from build123d import *

# Parameters (mm, degrees)
SKETCH1_R           = 17.5
BOSS_EXTRUDE1_DEPTH = 20
SKETCH2_R           = 21.5
BOSS_EXTRUDE2_DEPTH = 3
SKETCH3_W           = 19
SKETCH3_H           = 8.5
CUT_EXTRUDE3_DEPTH  = 23
FILLET11_R          = 4
FILLET12_R          = 4


with BuildPart() as part:
    # Sketch1 → Boss-Extrude1 (new body)
    with BuildSketch(Plane(origin=(0, 0, 0), x_dir=(1, 0, 0), z_dir=(0, 1, 0))):
        with Locations(Location((0, 0, 0), (0, 0, 270))):
            Circle(SKETCH1_R)
    extrude(amount=BOSS_EXTRUDE1_DEPTH)

    # Sketch2 → Boss-Extrude2 (add)
    with BuildSketch(Plane(origin=(0, 20, 0), x_dir=(1, 0, 0), z_dir=(0, 1, 0))):
        with Locations(Location((0, 0, 0), (0, 0, 270))):
            Circle(SKETCH2_R)
    extrude(amount=BOSS_EXTRUDE2_DEPTH)

    # Sketch3 → Cut-Extrude3 (cut)
    with BuildSketch(Plane(origin=(0, 23, 0), x_dir=(1, 0, 0), z_dir=(0, 1, 0))):
        with Locations((0, 0.083811037)):
            Rectangle(SKETCH3_W, SKETCH3_H)
        with Locations((0, 10.083811037)):
            Rectangle(SKETCH3_W, SKETCH3_H)
        with Locations((0, -9.916188963)):
            Rectangle(SKETCH3_W, SKETCH3_H)
    extrude(amount=-CUT_EXTRUDE3_DEPTH, mode=Mode.SUBTRACT)

    # Fillet11
    fillet11_edges = [part.edges().sort_by_distance(p)[0] for p in [
        (9.5, 11.5, 4.166188963),
        (-9.5, 11.5, 4.166188963),
        (-9.5, 11.5, -4.333811037),
        (9.5, 11.5, -4.333811037),
        (9.5, 11.5, 14.166188963),
        (-9.5, 11.5, 14.166188963),
        (-9.5, 11.5, 5.666188963),
        (9.5, 11.5, 5.666188963),
    ]]
    fillet(fillet11_edges, radius=FILLET11_R)

    # Fillet12
    fillet12_edges = [part.edges().sort_by_distance(p)[0] for p in [
        (9.5, 11.5, -14.333811037),
        (9.5, 11.5, -5.833811037),
        (-9.5, 11.5, -5.833811037),
        (-9.5, 11.5, -14.333811037),
    ]]
    fillet(fillet12_edges, radius=FILLET12_R)


solid = part.part
Read the model definition and answer for the solid it produces. Units are mm, in the model's axes. A direction names the side the tool comes from. Coordinates: 2 decimals unless noted, no trailing zeros. Order: outer loops, then holes, each group sorted by start corner. A loop starts at its lowest first (then second) coordinate and runs counter-clockwise, first axis right, second up. Notation, with made-up numbers: (18, -9.5) - (36, -9.5) arc R30 ccw to (36, 25.5) - close; hole circle Ø6 at (85, 86.5). An arc over 180 degrees is marked (long way). Use one line per item in the form item = value.
(1) Section C-C, the plane z = -11.5 is taken. Give the vertices of the cut face in (x, y).
Computed values:
outline = (-18.17, 20) - (-13.19, 20) - (-13.19, 0) - (-9.33, 0) - (-9.33, 23) - (-18.17, 23) - close; (9.33, 0) - (13.19, 0) - (13.19, 20) - (18.17, 20) - (18.17, 23) - (9.33, 23) - close
(2) Given pin 1 Ø3.5 at (x, y) = (-2, 11.5) entering from +Z; pin 2 Ø2 at (y, z) = (14, -9.5) entering from -X; pin 3 Ø0.6 at (y, z) = (12.5, 10) entering from +X, each flat-ended and moving along its own axis, determine where each tip first touches the part or whether it passes through.
Computed values:
pin_1 = 17.5
pin_2 = -15.3
pin_3 = 14.57
(3) Which of the six approach directions +Z, -Z, +X, -X, +Y, -Y give full straight-line access (tool end or side, diameter ignored) to faces 1 (the face through (-17.4, 20, 3.1)), 2 (the face through (0, 23, -5)), 3 (the face through (-8.297, 11.339, 13.026))?
Computed values:
face_1 = -Y
face_2 = +Z, -Z, +X, -X, +Y
face_3 = +Y, -Y
(4) Straight lines are drawn through the part: L1, parallel to Z at x = -6, y = 1.25; L2, parallel to Z at x = 1, y = 21.75; L3, parallel to Y at x = 19, z = 9.5. For each, find the intervals that lie inside material, in ascending order.
Computed values:
L1 = -16.44 to -14.3, -5.87 to -4.3, 4.13 to 5.7, 14.13 to 16.44
L2 = -21.48 to -14.33, -5.83 to -4.33, 4.17 to 5.67, 14.17 to 21.48
L3 = 20 to 23
(5) Section B-B, the plane y = 6.5 is taken. Give the vertices of the cut face in (x, z), then the cut area to 3 significant figures.
Computed values:
outline = circle Ø35 at (0, 0); hole (-9.5, -10.33) arc R4 ccw to (-5.5, -14.33) - (5.5, -14.33) arc R4 ccw to (9.5, -10.33) - (9.5, -9.83) arc R4 ccw to (5.5, -5.83) - (-5.5, -5.83) arc R4 ccw to (-9.5, -9.83) - close; hole (-9.5, -0.33) arc R4 ccw to (-5.5, -4.33) - (5.5, -4.33) arc R4 ccw to (9.5, -0.33) - (9.5, 0.17) arc R4 ccw to (5.5, 4.17) - (-5.5, 4.17) arc R4 ccw to (-9.5, 0.17) - close; hole (-9.5, 9.67) arc R4 ccw to (-5.5, 5.67) - (5.5, 5.67) arc R4 ccw to (9.5, 9.67) - (9.5, 10.17) arc R4 ccw to (5.5, 14.17) - (-5.5, 14.17) arc R4 ccw to (-9.5, 10.17) - close
area = 519 mm²
(6) Section D-D, the plane x = -8 is taken. Give the vertices of the cut face in (y, z).
Computed values:
outline = (0, -15.56) - (20, -15.56) - (20, -19.96) - (23, -19.96) - (23, -13.46) - (0, -13.46) - close; (0, -6.71) - (23, -6.71) - (23, -3.46) - (0, -3.46) - close; (0, 3.29) - (23, 3.29) - (23, 6.54) - (0, 6.54) - close; (0, 13.29) - (23, 13.29) - (23, 19.96) - (20, 19.96) - (20, 15.56) - (0, 15.56) - close
(7) Section A-A, the plane x = 0 is taken. Give the vertices of the cut face in (y, z).
Computed values:
outline = (0, -17.5) - (20, -17.5) - (20, -21.5) - (23, -21.5) - (23, -14.33) - (0, -14.33) - close; (0, -5.83) - (23, -5.83) - (23, -4.33) - (0, -4.33) - close; (0, 4.17) - (23, 4.17) - (23, 5.67) - (0, 5.67) - close; (0, 14.17) - (23, 14.17) - (23, 21.5) - (20, 21.5) - (20, 17.5) - (0, 17.5) - close
(8) For a pull along X with two mould halves and no side action, classify faces 4 (the face through (0, 12, -4.334)), 5 (the face through (14.531, 21.479, -15.846)), 6 (the face through (-8, 0, 4)) as pulls with the +X half, pulls with the -X half, needs draft (parallel to the pull), parting line crosses it, or undercut.
Computed values:
face_4 = undercut
face_5 = parting line crosses it
face_6 = needs draft
